from build123d import *

# Parameters (mm, degrees)
F1_DEPTH    = 15
F2_T1_DEPTH = 22.7150489639
F2_T3_DEPTH = 20.8646002419
F3_SIZE     = 1.99999


# Not quite as in the source:
# - a fillet or chamfer that OpenCascade refuses, or shapes differently, is made with other operations: its cross-section is extruded or revolved along the edge and cut away or added
# - a fillet or chamfer is up to 0.001 mm smaller than in the source, because OpenCascade refuses the exact size


with BuildPart() as f1:
    # F0 (on Top) → F1 (new body)
    with BuildSketch(Plane.XY):
        Polygon((0, 16), (0, 0), (-30, 0), (-30, -2.3844742682), (-30, -16.3243375719), (-28.4316577017, -16.3243375719), (-21.5928480029, -9.9000008777), (-21.5928480029, -7.5513185002), (-12.7507485449, -2.3844742682), (3, -2.3844742682), (28.4, 5.0389636308), (28.4, 18.6757165939), (23.4, 18.6757165939), (23.4, 8.0389636308), (3, 8.0389636308), (3, 18), (-27, 18), (-27, 16), align=None)
        Polygon((-28.5007357597, -13.9756565914), (-28.5007357597, -10.7289487496), (-28.5007357597, -9.9000008777), (-24.1621347258, -9.9000008777), align=None, mode=Mode.SUBTRACT)
        Polygon((-27.9481057078, -3.890137421), (-19.4514021277, -3.890137421), (-25.8757378906, -7.5513185002), (-27.9481057078, -7.5513185002), align=None, mode=Mode.SUBTRACT)
        Polygon((3, 5.0389636308), (20.7205470651, 5.0389636308), (3, 0), align=None, mode=Mode.SUBTRACT)
    extrude(amount=F1_DEPTH)

    # F2: chamfer of 1.5 on 2 edges, made by hand

    # F2_s2 → F2_t1 (cut)
    with BuildSketch(Plane.XY.offset(-3.8575244819)):
        Polygon((1.5, 18), (3, 16.5), (3, 18), align=None)
    extrude(amount=F2_T1_DEPTH, mode=Mode.SUBTRACT)

    # F2_s4 → F2_t3 (cut)
    with BuildSketch(Plane.XY.offset(-2.932300121)):
        Polygon((28.4, 6.163321624), (27.3207889969, 4.7235519827), (28.4, 5.0389636308), align=None)
    extrude(amount=F2_T3_DEPTH, mode=Mode.SUBTRACT)

    # F3 (size 2 in the source; OpenCascade refuses exactly that, so slightly less here)
    f3_edges = [f1.edges().sort_by_distance(p)[0] for p in [
        (-27, 18, 7.5),
    ]]
    chamfer(f3_edges, length=F3_SIZE)


solid = f1.part
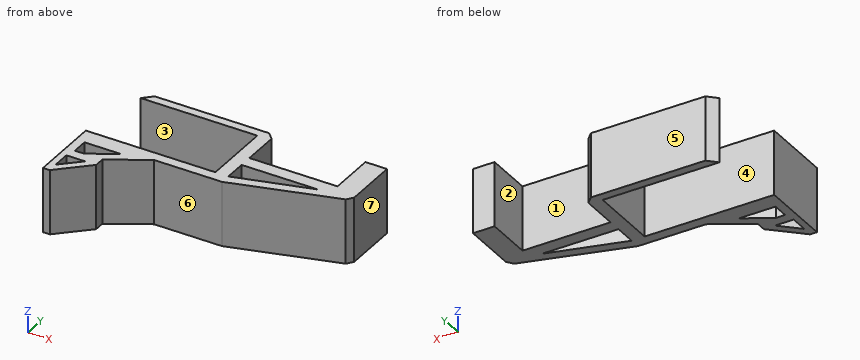
Build history of the part. All positions in model axes, mm. Face numbers are marked on the shaded views. A direction names the side the tool comes from. Round coordinates to 2 decimals unless told otherwise and drop trailing zeros. Write each loop counter-clockwise with the first axis right and the second up, starting at its lowest first coordinate (ties: lowest second). Pieces come first, ordered by that corner, then holes. Notation, with made-up numbers: (14.25, 57) -> (42.25, 57) arc R20 ccw to (42.25, 84) -> close; hole circle Ø3 at (-14, -28.5). An arc over 180 degrees is marked (long way). Write item = value, one per line.
(1) Band-saw the part on A-A (x = -5.5). Give the cut face in (y, z).
Answer:
outline = (-2.38, 0) -> (0, 0) -> (0, 15) -> (-2.38, 15) -> close; (16, 0) -> (18, 0) -> (18, 15) -> (16, 15) -> close
(2) Tool access for the marked faces 4, 5, 6 and 7: list every direction of +Z, -Z, +X, -X, +Y, -Y with a clear straight run to the whole face (end or side of a thin tool).
Answer:
face_4 = +Z, -Z, -X
face_5 = +Z, -Z, -X, +Y
face_6 = +Z, -Z, +X, -Y
face_7 = +Z, -Z, +X, +Y, -Y
(3) Flat gauge pins, fed straight in: pin 1 (4.5 mm diameter, centred on x = -7.5, z = 7, fed in from -Y); pin 2 (4.5 mm diameter, centred on x = 12, z = 7.5, fed in from +Y); pin 3 (7.5 mm diameter, centred on x = -7.5, z = 6, fed in from +Y). Where does each tip first touch, or does it go through?
Answer:
pin_1 = -2.38
pin_2 = 8.04
pin_3 = 18
(4) Band-saw the part on C-C (y = 10). Give the cut face in (x, z).
Answer:
outline = (0, 0) -> (3, 0) -> (3, 15) -> (0, 15) -> close; (23.4, 0) -> (28.4, 0) -> (28.4, 15) -> (23.4, 15) -> close
(5) Two-plate mould, pull along Y, no slides. Class the marked faces 1, 2 and 3: pulls with the +Y half, pulls with the -Y half, needs draft (parallel to the pull), parting line crosses it, or undercut.
Answer:
face_1 = pulls with the +Y half
face_2 = needs draft
face_3 = undercut
(6) Band-saw the part on B-B (z = 7). State how many separate pieces and enclosed holes the cut face has, then the cut area to 3 significant figures.
Answer:
separate_pieces = 1
enclosed_holes = 3
area = 452 mm2
(7) Probe L1, parallel to Y at x = -24, z = 12.5; L2, parallel to Y at x = -7, z = 5.5; L3, parallel to Y at x = -22.5, z = 4. List the from-to ranges inside material, lowest first.
Answer:
L1 = -12.16 to -6.48, -3.89 to 0, 16 to 18
L2 = -2.38 to 0, 16 to 18
L3 = -10.75 to -5.63, -3.89 to 0, 16 to 18
(8) Band-saw the part on D-D (x = -21). Give the cut face in (y, z), then the cut area to 3 significant figures.
Answer:
outline = (-7.2, 0) -> (-4.77, 0) -> (-4.77, 15) -> (-7.2, 15) -> close; (-3.89, 0) -> (0, 0) -> (0, 15) -> (-3.89, 15) -> close; (16, 0) -> (18, 0) -> (18, 15) -> (16, 15) -> close
area = 125 mm2
